```python
from build123d import *

# Parameters (mm, degrees)
BOSS_EXTRUDE1_DEPTH   = 8.5
SKETCH2_W             = 17
SKETCH2_H             = 17
CUT_EXTRUDE1_DEPTH    = 6
CUT_EXTRUDE2_REACH    = 5
CORTE_EXTRUS_O1_REACH = 22
ESBO_O1_R             = 2.7
CORTE_EXTRUS_O2_DEPTH = 1.5


with BuildPart() as part:
    # Sketch1 → Boss-Extrude1 (new body, symmetric)
    with BuildSketch(Plane(origin=(0, 0, 0), x_dir=(0, 0, -1), z_dir=(1, 0, 0))):
        Polygon((0, 0), (-20, 0), (-20, -3), (-11.5, -11.5), (-3, -20), (0, -20), align=None)
    extrude(amount=BOSS_EXTRUDE1_DEPTH, both=True)

    # Sketch2 → Cut-Extrude1 (cut, symmetric)
    with BuildSketch(Plane(origin=(0, 0, 0), x_dir=(0, 0, -1), z_dir=(1, 0, 0))):
        with Locations((-11.5, -11.5)):
            Rectangle(SKETCH2_W, SKETCH2_H)
    extrude(amount=CUT_EXTRUDE1_DEPTH, both=True, mode=Mode.SUBTRACT)

    # Sketch3 → Cut-Extrude2 (cut, up to next)
    with BuildSketch(Plane.XY.offset(3), mode=Mode.PRIVATE) as cut_extrude2_sk1:
        with BuildLine():
            Line((-3, -9), (-3, -12))
            ThreePointArc((-3, -12), (0, -15), (3, -12))
            Line((3, -12), (3, -9))
            ThreePointArc((3, -9), (0, -6), (-3, -9))
        make_face()
    cut_extrude2_tool1 = extrude(cut_extrude2_sk1.sketch, amount=-CUT_EXTRUDE2_REACH, mode=Mode.PRIVATE) & part.part
    add(cut_extrude2_tool1.solids().sort_by_distance((0, -10.5, 3))[0], mode=Mode.SUBTRACT)

    # Esboço1 → Corte-extrusão1 (cut, up to next)
    with BuildSketch(Plane(origin=(0, 0, 0), x_dir=(1, 0, 0), z_dir=(0, 1, 0)), mode=Mode.PRIVATE) as corte_extrus_o1_sk1:
        with Locations((0, -10.5)):
            Circle(ESBO_O1_R)
    corte_extrus_o1_tool1 = extrude(corte_extrus_o1_sk1.sketch, amount=-CORTE_EXTRUS_O1_REACH, mode=Mode.PRIVATE) & part.part
    add(corte_extrus_o1_tool1.solids().sort_by_distance((0, 0, 10.5))[0], mode=Mode.SUBTRACT)

    # Esboço3 → Corte-extrusão2 (cut)
    with BuildSketch(Plane.XZ.offset(3)):
        Polygon((0, 14.7), (-2.424871131, 14.7), (-3.637306696, 12.6), (-4.849742261, 10.5), (-3.637306696, 8.4), (-2.424871131, 6.3), (0, 6.3), (2.424871131, 6.3), (3.637306696, 8.4), (4.849742261, 10.5), (3.637306696, 12.6), (2.424871131, 14.7), align=None)
    extrude(amount=-CORTE_EXTRUS_O2_DEPTH, mode=Mode.SUBTRACT)


solid = part.part
```
Geometry check sheet. Reference: the model listing, model coordinates, mm. A direction names the side the tool comes from. Coordinates: 2 decimals unless noted, no trailing zeros. Order: outer loops, then holes, each group sorted by start corner. A loop starts at its lowest first (then second) coordinate and runs counter-clockwise, first axis right, second up. Notation, with made-up numbers: (41.5, 7.25) - (82.5, 7.25) arc R20 cw to (82.5, 39.25) - close; hole circle Ø5 at (29.25, 81.5). An arc over 180 degrees is marked (long way). Answer in a Markdown table with one row per item. Add a question column.
1. Gauge pin test, flat ends, axial feed: pin 1 Ø4 at (x, z) = (6, 9.5) entering from -Y; pin 2 Ø2.5 at (x, z) = (-1.5, 12) entering from -Y; pin 3 Ø3 at (x, z) = (-5.5, 14) entering from -Y. Record the tip position at first contact, or that the pin passes through.
2. Section check D-D (z = 18.5). Enter the section's corners in (x, y), plus the area to 3 significant figures.
3. Section check C-C (y = -13.75). Enter the section's corners in (x, z), plus the area to 3 significant figures.
4. Section check B-B (x = -0.5). Enter the section's corners in (y, z), plus the area to 3 significant figures.
5. Material ranges on L1, parallel to X at y = -1, z = 10.5; L2, parallel to Z at x = -1.5, y = -1.75; L3, parallel to X at y = -5.25, z = 7.5, recorded low to high. Write a range as [from, to].
6. Section check A-A (z = 1.5). Enter the section's corners in (x, y).
7. Access from +Z, -Z, +X, -X, +Y, -Y to the whole of each face (thin tool, end or side, straight path). Record for faces 1 (the face through (-4, -10, 0)), 2 (the face through (-6, -8, 8)), 3 (the face through (3.654, -2.26, 12.571)), 4 (the face through (3, -11, 2)).
8. Draft check along Z on faces 5 (the face through (-8.5, -8, 8)), 6 (the face through (3.62, -2.26, 8.37)), 7 (the face through (-0.1, -1.5, 13.4)), 8 (the face through (3, -14, 3)). Enter one of: +Z half, -Z half, draft (parallel to the pull), parting line (faces both ways), or undercut.
Data:
| question | item | result |
|---|---|---|
| 1 | pin 1 | stops at y = -15.5 |
| 1 | pin 2 | stops at y = -1.5 |
| 1 | pin 3 | stops at y = -10.41 |
| 2 | outline | (-8.5, -4.5) - (-6, -4.5) - (-6, -3) - (6, -3) - (6, -4.5) - (8.5, -4.5) - (8.5, 0) - (-8.5, 0) - close |
| 2 | area | 58.5 mm² |
| 3 | outline | (-8.5, 0) - (-2.44, 0) - (-2.44, 3) - (-6, 3) - (-6, 9.25) - (-8.5, 9.25) - close; (2.44, 0) - (8.5, 0) - (8.5, 9.25) - (6, 9.25) - (6, 3) - (2.44, 3) - close |
| 3 | area | 67.6 mm² |
| 4 | outline | (-20, 0) - (-14.96, 0) - (-14.96, 3) - (-20, 3) - close; (-6.04, 0) - (0, 0) - (0, 7.85) - (-1.5, 7.85) - (-1.5, 6.3) - (-3, 6.3) - (-3, 3) - (-6.04, 3) - close; (-3, 14.7) - (-1.5, 14.7) - (-1.5, 13.15) - (0, 13.15) - (0, 20) - (-3, 20) - close |
| 4 | area | 63.7 mm² |
| 5 | L1 | x = [-8.5, -2.7], [2.7, 8.5] |
| 5 | L2 | z = [0, 6.3], [14.7, 20] |
| 5 | L3 | x = [-8.5, -6], [6, 8.5] |
| 6 | outline | (-8.5, -20) - (8.5, -20) - (8.5, 0) - (-8.5, 0) - close; hole (-3, -12) arc R3 ccw to (3, -12) - (3, -9) arc R3 ccw to (-3, -9) - close |
| 7 | face 1 | -Z, +X, -X, +Y, -Y |
| 7 | face 2 | +Z, -Y |
| 7 | face 3 | -Y |
| 7 | face 4 | +Z, -Z |
| 8 | face 5 | draft |
| 8 | face 6 | undercut |
| 8 | face 7 | undercut |
| 8 | face 8 | +Z half |
